The drawing under review shows one solid part. Ordinate dimensions are in mm from its lowest x, y, z. Round coordinates to 2 decimals unless told otherwise and drop trailing zeros. Order: outer loops, then holes, each group sorted by start corner. A loop starts at its lowest first (then second) coordinate and runs counter-clockwise, first axis right, second up. Notation, with made-up numbers: (-38, -16.75) - (-3, -16.75) arc R9 ccw to (-3, -4.75) - close; hole circle Ø9 at (38.25, -13.75). An arc over 180 degrees is marked (long way). One line per question, with ' | ' between items.
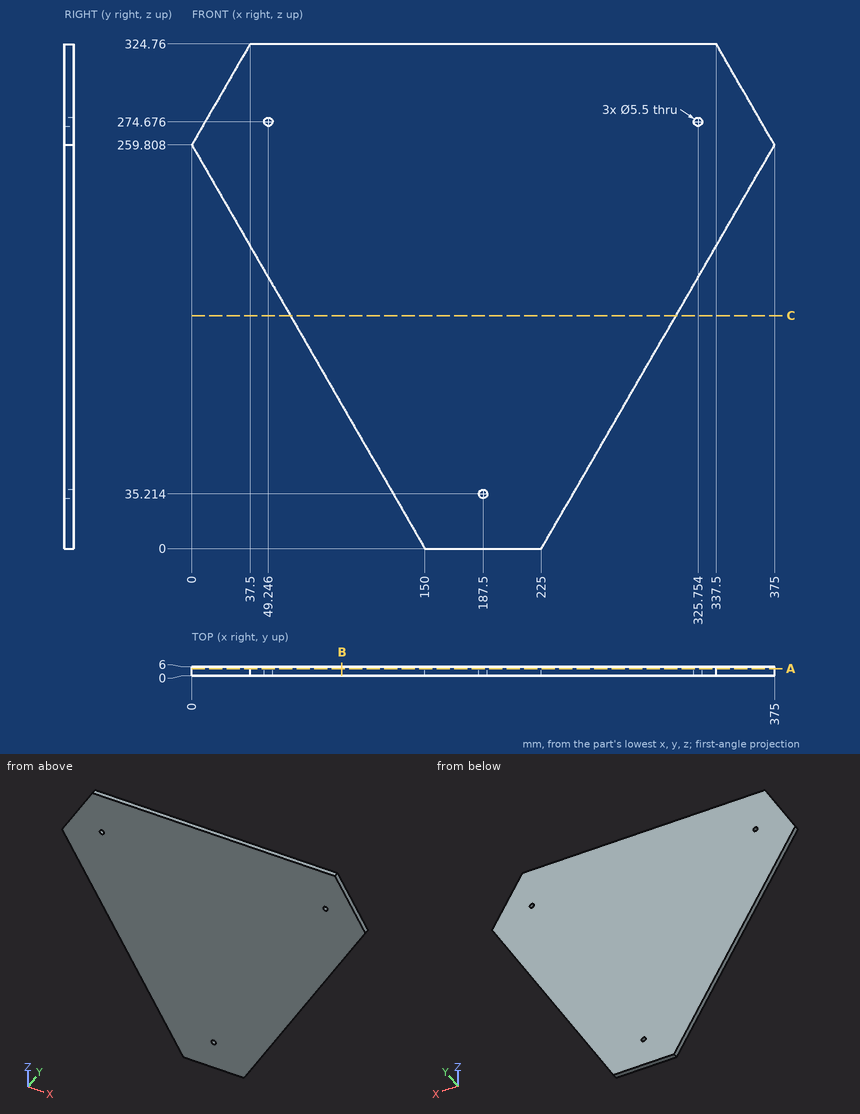
(1) We need section C-C on z = 150. State the section outline as (x, y) points, plus the area to 3 significant figures.
Output values:
outline: (63.4, 0) - (311.6, 0) - (311.6, 6) - (63.4, 6) - close | area: 1,490 mm^2
(2) We need section A-A on y = 4.75. Give the number of separate pieces and of enclosed holes in the cut face, plus the area to 3 significant figures.
Output values:
separate pieces: 1 | enclosed holes: 3 | area: 80,300 mm^2
(3) We need section B-B on x = 96.5. State the section outline as (y, z) points (1 decimal).
Output values:
outline: (0, 92.7) - (6, 92.7) - (6, 324.8) - (0, 324.8) - close
(4) Insertion check: pin 1 (10 mm diameter, centred on x = 123.5, z = 189, fed in from -Y); pin 2 (2 mm diameter, centred on x = 234.5, y = 2.5, fed in from -Z) (1 decimal); pin 3 (4.5 mm diameter, centred on x = 49.25, z = 274.68, fed in from +Y). Each pin has a flat end and moves straight along its axis. Give the tip position at first contact, or say it passes through.
Output values:
pin 1: y = 0 | pin 2: z = 14.7 | pin 3: through
(5) For probe 1 along Z at (x, y) = (28, 5.6) (1 decimal); probe 2 along Z at (x, y) = (234, 2.05) (1 decimal); probe 3 along X at (y, z) = (3.2, 84.5) (1 decimal), list the stretches that pass through material, from the lowest coordinate up. Write a range as [from, to].
Output values:
probe 1: [211.3, 308.3] | probe 2: [15.6, 324.8] | probe 3: [101.2, 273.8]
